```python
from build123d import *

# Parameters (mm, degrees)
SKETCH_1_W               = 330
SKETCH_1_H               = 60
EXTRUDE_1_DEPTH          = 10
FILLET_1_R               = 20
SKETCH_5_R               = 12.25
CUT_EXTRUDE_3_DEPTH      = 12
SKETCH_9_R               = 1.55
CUT_EXTRUDE_6_DEPTH      = 169.002976164
SKETCH_11_R              = 4.25
CUT_EXTRUDE_8_DEPTH      = 169.002976164
CUT_EXTRUDE_11_DEPTH     = 169.002976164
SKETCH_16_R              = 1.7
CUT_EXTRUDE_12_DEPTH     = 169.002976164
PATTERN_CIRCULAR_1_COUNT = 6


with BuildPart() as part:
    # 草图1 → 凸台-拉伸1 (new body)
    with BuildSketch(Plane(origin=(0, 0, 0), x_dir=(1, 0, 0), z_dir=(0, 1, 0))):
        Rectangle(SKETCH_1_W, SKETCH_1_H)
    extrude(amount=EXTRUDE_1_DEPTH)

    # 圆角1
    fillet_1_edges = [part.edges().sort_by_distance(p)[0] for p in [
        (165, 5, 30),
        (-165, 5, 30),
        (-165, 5, -30),
        (165, 5, -30),
    ]]
    fillet(fillet_1_edges, radius=FILLET_1_R)

    # 草图5 → 切除-拉伸3 (cut)
    with BuildSketch(Plane(origin=(0, 10, 0), x_dir=(1, 0, 0), z_dir=(0, 1, 0))):
        with Locations(Location((135, 0, 0), (0, 0, 270))):
            Circle(SKETCH_5_R)
    extrude(amount=-CUT_EXTRUDE_3_DEPTH, mode=Mode.SUBTRACT)

    # 草图9 → 切除-拉伸6 (cut, through all)
    with BuildSketch(Plane.XZ):
        with Locations(Location((119.5, 15.5, 0), (0, 0, 270))):
            Circle(SKETCH_9_R)
        with Locations(Location((150.5, 15.5, 0), (0, 0, 270))):
            Circle(SKETCH_9_R)
        with Locations(Location((150.5, -15.5, 0), (0, 0, 270))):
            Circle(SKETCH_9_R)
        with Locations(Location((119.5, -15.5, 0), (0, 0, 270))):
            Circle(SKETCH_9_R)
    extrude(amount=-CUT_EXTRUDE_6_DEPTH, mode=Mode.SUBTRACT)

    # 草图11 → 切除-拉伸8 (cut, through all)
    with BuildSketch(Plane.XZ):
        with Locations(Location((-140, 0, 0), (0, 0, 270))):
            Circle(SKETCH_11_R)
    extrude(amount=-CUT_EXTRUDE_8_DEPTH, mode=Mode.SUBTRACT)

    # 草图15 → 切除-拉伸11 (cut, through all)
    with BuildSketch(Plane.XZ):
        with BuildLine():
            Line((-85, 12.5), (85, 12.5))
            ThreePointArc((85, 12.5), (97.5, 0), (85, -12.5))
            Line((85, -12.5), (-85, -12.5))
            ThreePointArc((-85, -12.5), (-97.5, 0), (-85, 12.5))
        make_face()
    extrude(amount=-CUT_EXTRUDE_11_DEPTH, mode=Mode.SUBTRACT)

    # 草图16 → 切除-拉伸12 (cut, through all)
    with BuildSketch(Plane.XZ):
        with Locations(Location((-149, 0, 0), (0, 0, 270))):
            Circle(SKETCH_16_R)
    cut_extrude_12 = extrude(amount=-CUT_EXTRUDE_12_DEPTH, mode=Mode.SUBTRACT)

    # 阵列(圆周)1: 切除-拉伸12 ×6 about axis
    pattern_circular_1_axis = Axis((-140, 0, 0), (0, 1, 0))
    for i in range(1, PATTERN_CIRCULAR_1_COUNT):
        add(cut_extrude_12.rotate(pattern_circular_1_axis, i * 360 / PATTERN_CIRCULAR_1_COUNT), mode=Mode.SUBTRACT)


solid = part.part
```
Check sheet for the modelled part. Datum: model origin and axes. Units: mm. A direction names the side the tool comes from. Coordinates: 2 decimals unless noted, no trailing zeros. Loops run counter-clockwise (first coordinate to the right, second up) from the corner with the lowest first, then second, coordinate; pieces in that order, holes last. Notation, with made-up numbers: M -15,89 L 23,89 A27 ccw 23,105 Z; hole C 41.5,-15 d3. An arc over 180 degrees is marked long. Answer as a JSON object with one key per item and string values.
1. Sectioned sample at A-A on x = -140. Record the cut outline in (y, z).
Outcome:
{"outline": "M 0,-30 L 10,-30 L 10,-4.25 L 0,-4.25 Z; M 0,4.25 L 10,4.25 L 10,30 L 0,30 Z"}
2. Access from +Z, -Z, +X, -X, +Y, -Y to the whole of each face (thin tool, end or side, straight path). Record for faces 1 (the cylindrical face through (-97.497, 4.93, -0.275)), 2 (the cylindrical face through (158.986, 5.07, 24.297)).
Outcome:
{"face 1": "+Y, -Y", "face 2": "+Z, +X, +Y, -Y"}
3. Sectioned sample at C-C on x = -46.5. Record the cut outline in (y, z).
Outcome:
{"outline": "M 0,-30 L 10,-30 L 10,-12.5 L 0,-12.5 Z; M 0,12.5 L 10,12.5 L 10,30 L 0,30 Z"}
4. Release check for a two-part mould opening along Z. For faces 3 (the flat face through (-2, 5, 30)), 4 (the flat face through (-165, 5, 0)), 5 (the cylindrical face through (159.297, 5.07, -23.986)), 6 (the cylindrical face through (97.497, 4.93, 0.275)) record: pulls with the +Z half, pulls with the -Z half, needs draft (parallel to the pull), parting line crosses it, or undercut.
Outcome:
{"face 3": "pulls with the +Z half", "face 4": "needs draft", "face 5": "pulls with the -Z half", "face 6": "undercut"}
5. Depth check by flat-ended pin: P1, Ø2, axis at x = -135.5, z = 7.79, coming from the +Y side; P2, Ø4, axis at x = -149, z = 0, coming from the +Y side. Enter the tip coordinate at first touch or a pass-through.
Outcome:
{"P1": "through", "P2": "y = 10"}
6. Sectioned sample at B-B on y = 2.25. Count the separate pieces of the cut face and the enclosed holes in it, and give its area (3 significant figures).
Outcome:
{"separate pieces": "1", "enclosed holes": "13", "area": "14,100 mm²"}
7. Scan lines: L1, parallel to Z at x = -66.5, y = 3; L2, parallel to X at y = 8.5, z = 10.5; L3, parallel to X at y = 1.25, z = 2.5. Record each from-to range of solid material in increasing order. Write a range as from..to.
Outcome:
{"L1": "-30..-12.5, 12.5..30", "L2": "-164.99..-91.78, 91.78..128.69, 141.31..164.99", "L3": "-165..-143.44, -136.56..-97.25, 97.25..123.01, 146.99..165"}
